The listing builds one solid part. Answer for the finished solid, in the listing's coordinates (mm). Give positions to 0.01 mm unless a question says otherwise; leave off trailing zeros. Order: outer loops, then holes, each group sorted by start corner. A loop starts at its lowest first (then second) coordinate and runs counter-clockwise, first axis right, second up.
```python
from build123d import *

# Parameters (mm, degrees)
SKETCH1_W           = 25.4
SKETCH1_H           = 50.8
SKETCH1_W_2         = 22.225
SKETCH1_H_2         = 47.625
BOSS_EXTRUDE1_DEPTH = 254
SKETCH2_R           = 14.2875
CUT_EXTRUDE1_DEPTH  = 257.527425434


with BuildPart() as part:
    # Sketch1 → Boss-Extrude1 (new, symmetric)
    with BuildSketch(Plane.XY):
        Rectangle(SKETCH1_W, SKETCH1_H)
        Rectangle(SKETCH1_W_2, SKETCH1_H_2, mode=Mode.SUBTRACT)
    extrude(amount=BOSS_EXTRUDE1_DEPTH, both=True)

    # Sketch2 → Cut-Extrude1 (cut, through all)
    with BuildSketch(Plane(origin=(12.7, 0, 0), x_dir=(0, 0, -1), z_dir=(1, 0, 0))):
        with Locations((224.210207487, 0)):
            Circle(SKETCH2_R)
    extrude(amount=-CUT_EXTRUDE1_DEPTH, mode=Mode.SUBTRACT)


solid = part.part
```
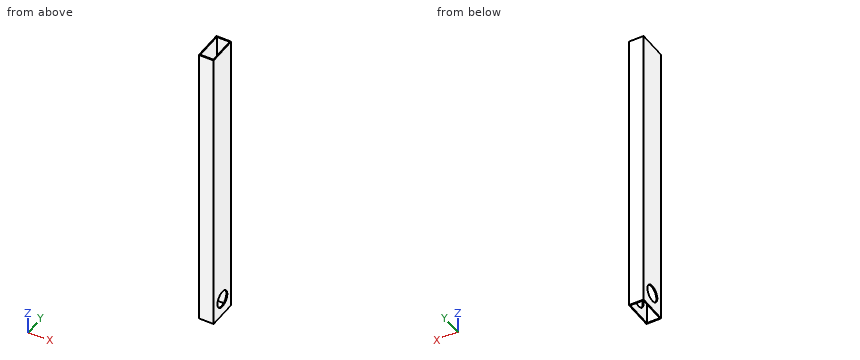
1) Find section A-A (y = 0). Write down the section's boundary in (x, z), then the cut area to 3 significant figures.
Geometry says:
outline: (-12.7, -254) - (-11.11, -254) - (-11.11, -238.5) - (-12.7, -238.5) - close; (-12.7, -209.92) - (-11.11, -209.92) - (-11.11, 254) - (-12.7, 254) - close; (11.11, -254) - (12.7, -254) - (12.7, -238.5) - (11.11, -238.5) - close; (11.11, -209.92) - (12.7, -209.92) - (12.7, 254) - (11.11, 254) - close
area: 1,520 mm2
2) Find section D-D (y = -19.5). Write down the section's boundary in (x, z), then the cut area to 3 significant figures.
Geometry says:
outline: (-12.7, -254) - (-11.11, -254) - (-11.11, 254) - (-12.7, 254) - close; (11.11, -254) - (12.7, -254) - (12.7, 254) - (11.11, 254) - close
area: 1,610 mm2
3) Find section C-C (z = -51.5). Write down the section's boundary in (x, y).
Geometry says:
outline: (-12.7, -25.4) - (12.7, -25.4) - (12.7, 25.4) - (-12.7, 25.4) - close; hole (-11.11, -23.81) - (11.11, -23.81) - (11.11, 23.81) - (-11.11, 23.81) - close
4) Straight lines are drawn through the part: probe 1 along Y at (x, z) = (-9, -172); probe 2 along X at (y, z) = (11, -56); probe 3 along Z at (x, y) = (11.25, 1.5). For each, find the intervals that lie inside material, in ascending order.
Geometry says:
probe 1: y = -25.4 to -23.81, 23.81 to 25.4
probe 2: x = -12.7 to -11.11, 11.11 to 12.7
probe 3: z = -254 to -238.42, -210 to 254
5) Find section B-B (x = 0). Write down the section's boundary in (y, z), then the cut area to 3 significant figures.
Geometry says:
outline: (-25.4, -254) - (-23.81, -254) - (-23.81, 254) - (-25.4, 254) - close; (23.81, -254) - (25.4, -254) - (25.4, 254) - (23.81, 254) - close
area: 1,610 mm2
